Work out the finished part from the listing and answer in its coordinate system (mm). A direction names the side the tool comes from. Coordinates: 2 decimals unless noted, no trailing zeros. Loops run counter-clockwise (first coordinate to the right, second up) from the corner with the lowest first, then second, coordinate; pieces in that order, holes last. Notation, with made-up numbers: (27, 70) - (86, 70) arc R23 ccw to (86, 105) - close; hole circle Ø8 at (76, 50.5). An arc over 180 degrees is marked (long way). Write each question's results on one line, items separated by ' | '. Start each with the question number.
1. A cutting plane is placed at C-C on y = 0.9. Determine the outline of the cut face in (x, z).
2. Which of the six approach directions +Z, -Z, +X, -X, +Y, -Y give full straight-line access (tool end or side, diameter ignored) to faces 1 (the flat face through (-4, 0, 1)), 2 (the flat face through (0, 0, 0.4))?
3. This flat-tipped pin is pushed along its axis until it touches: P1, Ø2, axis at x = 1, y = 0.5, coming from the -Z side. Where does it stop, or does it pass through?
4. Find the intervals of material crossed by line 1 along Z through (x, y) = (-1, -0.25); line 2 along X through (y, z) = (-0.05, 0.6), in increasing order. Write a range as [from, to].
5. A cutting plane is placed at A-A on z = 0.6. Determine the outline of the cut face in (x, y), then the cut area to 3 significant figures.
6. Determine the mould class of faces 3 (the flat face through (4, 0, 1)), 4 (the flat face through (0, 0, 0.8)), 5 (the flat face through (0, 0, 1.2)) for opening direction Z: released by +Z, released by -Z, zero draft, split by the parting line, or undercut.
7. A cutting plane is placed at B-B on x = -2. Determine the outline of the cut face in (y, z), then the cut area to 3 significant figures.
from build123d import *

# Parameters (mm, degrees)
SKETCH2_W           = 8
SKETCH2_H           = 4
BOSS_EXTRUDE1_DEPTH = 0.4
SKETCH3_W           = 0.4
SKETCH3_H           = 4
BOSS_EXTRUDE2_DEPTH = 0.8
SKETCH4_W           = 0.4
SKETCH4_H           = 4
BOSS_EXTRUDE3_DEPTH = 0.8
BOSS_EXTRUDE4_REACH = 9.6
SKETCH5_W           = 0.4
SKETCH5_H           = 4


with BuildPart() as part:
    # Sketch2 → Boss-Extrude1 (new body)
    with BuildSketch(Plane.XY):
        Rectangle(SKETCH2_W, SKETCH2_H)
    extrude(amount=BOSS_EXTRUDE1_DEPTH)

    # Sketch3 → Boss-Extrude2 (add)
    with BuildSketch(Plane.XY.offset(0.4)):
        with Locations((-3.8, 0)):
            Rectangle(SKETCH3_W, SKETCH3_H)
    extrude(amount=BOSS_EXTRUDE2_DEPTH)

    # Sketch4 → Boss-Extrude3 (add)
    with BuildSketch(Plane.XY.offset(0.4)):
        with Locations((3.8, 0)):
            Rectangle(SKETCH4_W, SKETCH4_H)
    extrude(amount=BOSS_EXTRUDE3_DEPTH)

    # Sketch5 → Boss-Extrude4 (add, up to next)
    with BuildSketch(Plane(origin=(-3.6, 0, 0), x_dir=(0, 0, -1), z_dir=(1, 0, 0)), mode=Mode.PRIVATE) as boss_extrude4_sk1:
        with Locations((-1, 0)):
            Rectangle(SKETCH5_W, SKETCH5_H)
    boss_extrude4_tool1 = extrude(boss_extrude4_sk1.sketch, amount=BOSS_EXTRUDE4_REACH, mode=Mode.PRIVATE) - part.part
    add(boss_extrude4_tool1.solids().sort_by_distance((-3.6, 0, 1))[0])


solid = part.part
Values:
1) outline: (-4, 0) - (4, 0) - (4, 1.2) - (-4, 1.2) - close; hole (-3.6, 0.4) - (3.6, 0.4) - (3.6, 0.8) - (-3.6, 0.8) - close
2) face 1: +Z, -Z, -X, +Y, -Y | face 2: +Y, -Y
3) P1: z = 0
4) line 1: [0, 0.4], [0.8, 1.2] | line 2: [-4, -3.6], [3.6, 4]
5) outline: (-4, -2) - (-3.6, -2) - (-3.6, 2) - (-4, 2) - close; (3.6, -2) - (4, -2) - (4, 2) - (3.6, 2) - close | area: 3.20 mm^2
6) face 3: zero draft | face 4: undercut | face 5: released by +Z
7) outline: (-2, 0) - (2, 0) - (2, 0.4) - (-2, 0.4) - close; (-2, 0.8) - (2, 0.8) - (2, 1.2) - (-2, 1.2) - close | area: 3.20 mm^2
